The listing builds one solid part. Answer for the finished solid, in the listing's coordinates (mm). A direction names the side the tool comes from. Round coordinates to 2 decimals unless told otherwise and drop trailing zeros. Loops run counter-clockwise (first coordinate to the right, second up) from the corner with the lowest first, then second, coordinate; pieces in that order, holes last. Notation, with made-up numbers: (32.5, 57) -> (42.5, 57) arc R9 cw to (42.5, 72) -> close; hole circle Ø2 at (70, -33). An arc over 180 degrees is marked (long way). Answer in a Markdown table with one row per item. Add a question column.
Autodesk Inventor part; units mm, degrees
ref_plane "YZ Plane" through (0, 0, 0) normal (1, 0, 0) x (0, 1, 0)
ref_plane "XZ Plane" through (0, 0, 0) normal (0, 1, 0) x (-1, 0, 0)
ref_plane "XY Plane" through (0, 0, 0) normal (0, 0, 1) x (1, 0, 0)
sketch "Sketch1" plane through (0, 0, 0) normal (0, 1, 0) x (-1, 0, 0)
  line L0 (0, 0) -> (0, -14.0125) construction
  line L1 (12.3617, 25.4) -> (12.3617, -5.3655)
  line L2 (12.3617, -5.3655) -> (18.1749, -5.3655)
  line L3 (18.1844, -7.8927) -> (18.1844, -25.4)
  line L4 (18.1749, 25.4) -> (18.1749, 0.9638)
  line L5 (18.1749, 0.9638) -> (24.4214, 0.9638)
  line L6 (24.4214, 0.9638) -> (24.4214, -25.4)
  line L7 (18.1749, 25.4) -> (12.3617, 25.4)
  line L8 (18.1844, -25.4) -> (24.4214, -25.4)
  line L9 (-12.3617, 25.4) -> (-12.3617, -5.3655)
  line L10 (-12.3617, -5.3655) -> (-18.1749, 9.6342)
  line L11 (-18.1844, -7.8927) -> (-18.1844, -25.4)
  line L12 (-18.1749, 25.4) -> (-18.1749, 0.9638)
  line L13 (-18.1749, 0.9638) -> (-24.4214, 0.9638)
  line L14 (-24.4214, 0.9638) -> (-24.4214, -25.4)
  line L15 (-18.1749, 25.4) -> (-12.3617, 25.4)
  line L16 (-18.1844, -25.4) -> (-24.4214, -25.4)
  line L17 (12.3617, -5.3655) -> (18.1844, -7.8927)
  line L18 (-12.3617, -5.3655) -> (-18.1844, -7.8927)
  line L19 (12.3617, -5.3655) -> (0, 0) construction
  line L20 (27.1198, 0) -> (23.5153, 0) construction
  point P0 (18.1938, 0)
  point P1 (-18.1938, 0)
  point P2 (25.3175, 0)
  dimension "d10" = 50.8
  dimension "d11" = 25.4
extrude "Extrusion1" add sketch "Sketch1" against normal mid plane 25.4
sketch "Sketch2" plane through (0, -12.7, 0) normal (0, -1, 0) x (1, 0, 0)
  line L0 (-12.3617, -5.3655) -> (-12.3617, 25.4)
  line L1 (-12.3617, 25.4) -> (-18.1749, 25.4)
  line L2 (-18.1749, 25.4) -> (-18.1749, 0.9638)
  line L3 (-18.1749, 0.9638) -> (-24.4214, 0.9638)
  line L4 (-24.4214, 0.9638) -> (-24.4214, -25.4)
  line L5 (-24.4214, -25.4) -> (-18.1844, -25.4)
  line L6 (-18.1844, -25.4) -> (-18.1844, -7.8927)
  line L7 (24.4214, 0.9638) -> (18.1749, 0.9638)
  line L8 (18.1749, 0.9638) -> (18.1749, 25.4)
  line L9 (18.1749, 25.4) -> (12.3617, 25.4)
  line L10 (12.3617, 25.4) -> (12.3617, -5.3655)
  line L11 (18.1844, -7.8927) -> (18.1844, -25.4)
  line L12 (18.1844, -25.4) -> (24.4214, -25.4)
  line L13 (24.4214, -25.4) -> (24.4214, 0.9638)
  line L14 (18.1749, 25.4) -> (12.3617, 25.4)
  line L15 (-12.3617, 25.4) -> (-18.1749, 25.4)
  line L16 (18.1749, 25.4) -> (-18.1749, 25.4)
  line L17 (24.4214, 0.9638) -> (24.4214, -25.4)
  line L18 (24.4214, -25.4) -> (-24.4214, -25.4)
  line L19 (12.3617, -5.3655) -> (18.1844, -7.8927)
  line L20 (-18.1844, -7.8927) -> (-12.3617, -5.3655)
  point P0 (0, 0)
extrude "Extrusion2" add sketch "Sketch2" along normal blind 1.5875
sketch "Sketch4" plane through (0, -12.7, 0) normal (0, 1, 0) x (1, 0, 0)
  line L0 (18.1844, 7.8927) -> (18.1844, 25.4)
  line L1 (-18.1844, 25.4) -> (18.1844, 25.4)
  line L2 (-18.1844, 25.4) -> (-18.1844, 7.8927)
  line L3 (-18.1844, 7.8927) -> (-12.3617, 5.3655)
  line L4 (-12.3617, 5.3655) -> (-12.3617, -25.4)
  line L5 (12.3617, -25.4) -> (-12.3617, -25.4)
  line L6 (12.3617, -25.4) -> (12.3617, 5.3655)
  line L7 (12.3617, 5.3655) -> (18.1844, 7.8927)
  line L8 (-18.1844, 25.4) -> (18.1844, 25.4)
  line L9 (18.1844, 25.4) -> (18.1844, 23.7858)
  line L10 (18.1844, 23.7858) -> (-18.1844, 23.7858)
  line L11 (-18.1844, 23.7858) -> (-18.1844, 25.4)
  point P0 (0, 0)
extrude "Extrusion4" add sketch "Sketch4" along normal up to surface (25.4 mm away) contours L10 L2 L1 L0
properties part number "large_room1"
Item 1: Flat-ended cylindrical pins translate along their axes: P1, Ø2, axis at y = -7, z = 11, coming from the -X side; P2, Ø3, axis at x = 21.5, y = 5, coming from the +Z side; P3, Ø6, axis at x = 3, y = 0, coming from the +Z side. Find the tip coordinate at first contact, or state that the pin passes through.
Item 2: Section B-B, the plane x = -7 is taken. Write down the section's boundary in (y, z), and give its area (3 significant figures).
Item 3: Consider L1, parallel to X at y = 11.75, z = -1.5; L2, parallel to X at y = 6, z = 6; L3, parallel to Y at x = -6, z = 9.5. Determine where each line is inside the solid, lowest interval first. Write a range as from..to.
Item 4: For faces 1 (the flat face through (18.175, -1, 13)), 2 (the flat face through (-18.184, 0, -16)), 3 (the flat face through (-12.362, 0, 10)), 4 (the flat face through (-21, -1, 0.964)), determine the directions among +Z, -Z, +X, -X, +Y, -Y from which every point of the face is accessible in a straight line to the end or side of a thin tool.
Item 5: Section C-C, the plane y = -7.25 is taken. Write down the section's boundary in (x, z), and give its area (3 significant figures).
Item 6: The mould has two halves that part along Z. Classify faces 5 (the flat face through (21, -1, 0.964)), 6 (the flat face through (13, 12.7, -4)), 7 (the flat face through (18.184, 0, -16)): +Z half, -Z half, draft (parallel to the pull), parting line (faces both ways), or undercut.
Item 7: Section A-A, the plane z = 0 is taken. Write down the section's boundary in (x, y), and give its area (3 significant figures).
Item 8: Section D-D, the plane z = -8.5 is taken. Write down the section's boundary in (x, y), and give its area (3 significant figures).
Here are the results:
| question | item | result |
|---|---|---|
| 1 | P1 | stops at x = -18.17 |
| 1 | P2 | stops at z = 0.96 |
| 1 | P3 | stops at z = -23.79 |
| 2 | outline | (-14.29, -25.4) -> (12.7, -25.4) -> (12.7, -23.79) -> (-12.7, -23.79) -> (-12.7, 25.4) -> (-14.29, 25.4) -> close |
| 2 | area | 122 mm² |
| 3 | L1 | x = -24.42..-12.36, 12.36..24.42 |
| 3 | L2 | x = -18.17..-12.36, 12.36..18.17 |
| 3 | L3 | y = -14.29..-12.7 |
| 4 | face 1 | +Z, +X, +Y, -Y |
| 4 | face 2 | +Y |
| 4 | face 3 | +Z, +Y |
| 4 | face 4 | +Z, -X, +Y, -Y |
| 5 | outline | (-24.42, -25.4) -> (24.42, -25.4) -> (24.42, 0.96) -> (18.17, 0.96) -> (18.17, 25.4) -> (12.36, 25.4) -> (12.36, -5.37) -> (18.18, -7.89) -> (18.18, -23.79) -> (-18.18, -23.79) -> (-18.18, -7.89) -> (-12.36, -5.37) -> (-12.36, 25.4) -> (-18.17, 25.4) -> (-18.17, 0.96) -> (-24.42, 0.96) -> close |
| 5 | area | 760 mm² |
| 6 | face 5 | +Z half |
| 6 | face 6 | draft |
| 6 | face 7 | undercut |
| 7 | outline | (-24.42, -14.29) -> (24.42, -14.29) -> (24.42, 12.7) -> (12.36, 12.7) -> (12.36, -12.7) -> (-12.36, -12.7) -> (-12.36, 12.7) -> (-24.42, 12.7) -> close |
| 7 | area | 690 mm² |
| 8 | outline | (-24.42, -14.29) -> (24.42, -14.29) -> (24.42, 12.7) -> (18.18, 12.7) -> (18.18, -12.7) -> (-18.18, -12.7) -> (-18.18, 12.7) -> (-24.42, 12.7) -> close |
| 8 | area | 394 mm² |
